The listing builds one solid part. Answer for the finished solid, in the listing's coordinates (mm). A direction names the side the tool comes from. Give positions to 0.01 mm unless a question says otherwise; leave off trailing zeros. Loops run counter-clockwise (first coordinate to the right, second up) from the corner with the lowest first, then second, coordinate; pieces in that order, holes last. Notation, with made-up numbers: (-19.75, 9.5) -> (-11.75, 9.5) arc R18 cw to (-11.75, 36.5) -> close; hole circle Ø1 at (-8, 13). An arc over 180 degrees is marked (long way). One line per question, with ' | ' between items. Start each with the question number.
from build123d import *

# Parameters (mm, degrees)
ESQUISSE1_R             = 1
BOSS_EXTRU_1_DEPTH      = 5
ESQUISSE2_R             = 1.5
ENL_V_MAT_EXTRU_1_DEPTH = 6
ESQUISSE3_R             = 1.5
ENL_V_MAT_EXTRU_2_DEPTH = 6
ESQUISSE4_R             = 1.5
ENL_V_MAT_EXTRU_3_DEPTH = 6
ESQUISSE5_R             = 1.5
ENL_V_MAT_EXTRU_5_DEPTH = 6


with BuildPart() as part:
    # Esquisse1 → Boss.-Extru.1 (new body)
    with BuildSketch(Plane(origin=(0, 0, 0), x_dir=(1, 0, 0), z_dir=(0, 1, 0))):
        with BuildLine():
            Line((-120.5, 31.2), (120.5, 31.2))
            ThreePointArc((120.5, 31.2), (126.156854249, 28.856854249), (128.5, 23.2))
            Line((128.5, 23.2), (128.5, -219.467382599))
            ThreePointArc((128.5, -219.467382599), (126.772639772, -224.43266107), (122.336502426, -227.253733403))
            Line((122.336502426, -227.253733403), (48.443442049, -244.68228088))
            ThreePointArc((48.443442049, -244.68228088), (45.399263454, -245.077558471), (42.33836323, -244.8448408))
            ThreePointArc((42.33836323, -244.8448408), (33.490774319, -239.702526143), (30, -230.082873123))
            ThreePointArc((30, -230.082873123), (28.945508514, -222.073215083), (25.853895909, -214.609402001))
            Line((25.853895909, -214.609402001), (10.681549424, -188.330127019))
            Line((10.681549424, -188.330127019), (8.181549424, -184))
            ThreePointArc((8.181549424, -184), (-2.618897308, -173.730489766), (-16.376585234, -168))
            Line((-16.376585234, -168), (-33.623414766, -168))
            ThreePointArc((-33.623414766, -168), (-47.381102692, -173.730489766), (-58.181549424, -184))
            Line((-58.181549424, -184), (-60.681549424, -188.330127019))
            Line((-60.681549424, -188.330127019), (-75.853895909, -214.609402001))
            ThreePointArc((-75.853895909, -214.609402001), (-78.945508514, -222.073215083), (-80, -230.082873123))
            ThreePointArc((-80, -230.082873123), (-81.87001368, -237.335697347), (-87.013794564, -242.780137503))
            ThreePointArc((-87.013794564, -242.780137503), (-95.194460163, -245.081612578), (-103.312708305, -242.568820449))
            Line((-103.312708305, -242.568820449), (-124.933444429, -228.174488322))
            ThreePointArc((-124.933444429, -228.174488322), (-127.552217929, -225.292381715), (-128.5, -221.515316414))
            Line((-128.5, -221.515316414), (-128.5, 23.2))
            ThreePointArc((-128.5, 23.2), (-126.156854249, 28.856854249), (-120.5, 31.2))
        make_face()
        with Locations((41, -212.75)):
            Circle(ESQUISSE1_R, mode=Mode.SUBTRACT)
        with Locations((41, -240.25)):
            Circle(ESQUISSE1_R, mode=Mode.SUBTRACT)
        with Locations((-91, -212.75)):
            Circle(ESQUISSE1_R, mode=Mode.SUBTRACT)
        with Locations((-91, -240.25)):
            Circle(ESQUISSE1_R, mode=Mode.SUBTRACT)
    extrude(amount=-BOSS_EXTRU_1_DEPTH)

    # Esquisse2 → Enlèv. mat.-Extru.1 (cut, through all)
    with BuildSketch(Plane(origin=(0, 0, 0), x_dir=(1, 0, 0), z_dir=(0, 1, 0))):
        with Locations((-118.5, 11.2)):
            Circle(ESQUISSE2_R)
        with Locations((-25, -163)):
            Circle(ESQUISSE2_R)
        with Locations((118.5, 11.2)):
            Circle(ESQUISSE2_R)
        with Locations((118.5, -200.8)):
            Circle(ESQUISSE2_R)
        with Locations((-118.5, -200.8)):
            Circle(ESQUISSE2_R)
    extrude(amount=-ENL_V_MAT_EXTRU_1_DEPTH, mode=Mode.SUBTRACT)

    # Esquisse3 → Enlèv. mat.-Extru.2 (cut, through all)
    with BuildSketch(Plane(origin=(0, 0, 0), x_dir=(1, 0, 0), z_dir=(0, 1, 0))):
        with Locations((62, -140.8)):
            Circle(ESQUISSE3_R)
        with Locations((-62, -140.8)):
            Circle(ESQUISSE3_R)
        with Locations((62, -13.8)):
            Circle(ESQUISSE3_R)
        with Locations((-62, -13.8)):
            Circle(ESQUISSE3_R)
    extrude(amount=-ENL_V_MAT_EXTRU_2_DEPTH, mode=Mode.SUBTRACT)

    # Esquisse4 → Enlèv. mat.-Extru.3 (cut, through all)
    with BuildSketch(Plane(origin=(0, 0, 0), x_dir=(1, 0, 0), z_dir=(0, 1, 0))):
        with Locations((-35, -40)):
            Circle(ESQUISSE4_R)
        with Locations((35, -110)):
            Circle(ESQUISSE4_R)
    extrude(amount=-ENL_V_MAT_EXTRU_3_DEPTH, mode=Mode.SUBTRACT)

    # Esquisse5 → Enlèv. mat.-Extru.5 (cut, through all)
    with BuildSketch(Plane(origin=(0, 0, 0), x_dir=(1, 0, 0), z_dir=(0, 1, 0))):
        with Locations((61, -211.3)):
            Circle(ESQUISSE5_R)
        with Locations((99, -211.3)):
            Circle(ESQUISSE5_R)
        with Locations((99, -173.3)):
            Circle(ESQUISSE5_R)
        with Locations((61, -173.3)):
            Circle(ESQUISSE5_R)
        with BuildLine():
            Line((73, -177.3), (87, -177.3))
            ThreePointArc((87, -177.3), (92.656854249, -179.643145751), (95, -185.3))
            Line((95, -185.3), (95, -199.3))
            ThreePointArc((95, -199.3), (92.656854249, -204.956854249), (87, -207.3))
            Line((87, -207.3), (73, -207.3))
            ThreePointArc((73, -207.3), (67.343145751, -204.956854249), (65, -199.3))
            Line((65, -199.3), (65, -185.3))
            ThreePointArc((65, -185.3), (67.343145751, -179.643145751), (73, -177.3))
        make_face()
    extrude(amount=-ENL_V_MAT_EXTRU_5_DEPTH, mode=Mode.SUBTRACT)


solid = part.part
1. This flat-tipped pin is pushed along its axis until it touches: pin 1 Ø1.5 at (x, y) = (82, -2.5) entering from +Z. Where does it stop, or does it pass through?
2. For faces 1 (the cylindrical face through (126.8, -2.5, 224.4)), 2 (the cylindrical face through (-2.44, -2.46, 173.85)), 3 (the cylindrical face through (92.719, -2.465, 204.894)), determine the directions among +Z, -Z, +X, -X, +Y, -Y from which every point of the face is accessible in a straight line to the end or side of a thin tool.
3. The part is cut by section C-C (x = -50). Write down the section's boundary in (y, z), plus the area to 3 significant figures.
4. The part is cut by section D-D (x = 108). Write down the section's boundary in (y, z), plus the area to 3 significant figures.
5. The part is cut by section B-B (y = -3.7). Count the separate pieces of the cut face and the enclosed holes in it, plus the area to 3 significant figures.
6. Straight lines are drawn through the part: L1, parallel to Z at x = 118.5, y = -1.5; L2, parallel to X at y = -4, z = 140.8; L3, parallel to X at y = -3.4, z = 184. For each, find the intervals that lie inside material, in ascending order.
7. Determine the mould class of faces 4 (the cylindrical face through (-126.219, -2.465, -28.794)), 5 (the cylindrical face through (-47.21, -2.46, 173.62)), 6 (the cylindrical face through (67.281, -2.465, 179.706)) for opening direction Z: released by +Z, released by -Z, zero draft, split by the parting line, or undercut.
8. The part is cut by section A-A (x = 82). Write down the section's boundary in (y, z), plus the area to 3 significant figures.
Check sheet entries:
1) pin 1: stops at z = 236.94
2) face 1: +Z, +X, +Y, -Y | face 2: +Z, +Y, -Y | face 3: +Y, -Y
3) outline: (-5, -31.2) -> (0, -31.2) -> (0, 175.59) -> (-5, 175.59) -> close | area: 1,030 mm^2
4) outline: (-5, -31.2) -> (0, -31.2) -> (0, 230.64) -> (-5, 230.64) -> close | area: 1,310 mm^2
5) separate pieces: 1 | enclosed holes: 20 | area: 62,200 mm^2
6) L1: z = -31.2 to -12.7, -9.7 to 199.3, 202.3 to 228.16 | L2: x = -128.5 to -63.5, -60.5 to 60.5, 63.5 to 128.5 | L3: x = -128.5 to -58.18, 8.18 to 65.11, 94.89 to 128.5
7) face 4: released by -Z | face 5: released by +Z | face 6: undercut
8) outline: (-5, -31.2) -> (0, -31.2) -> (0, 177.3) -> (-5, 177.3) -> close; (-5, 207.3) -> (0, 207.3) -> (0, 236.77) -> (-5, 236.77) -> close | area: 1,190 mm^2
